```python
from build123d import *

# Parameters (mm, degrees)
SKETCH1_R            = 47
BASE_DEPTH           = 36.5
SKETCH2_W            = 38.1
SKETCH2_H            = 3.81
A_ARMS_DEPTH         = 38.1
FILLET_A_ARM_TAB_F_R = 20.32
FILLET2_R            = 50.8
SKETCH3_R            = 3.937
BOSS_EXTRUDE3_DEPTH  = 10
FILLET3_R            = 12.7
SKETCH6_R            = 3.81
TAB_HOLES_1_DEPTH    = 224.393667494
SKETCH7_R            = 3.81
TAB_HOLES_2_DEPTH    = 201.571915927
CUT_EXTRUDE2_DEPTH   = 154.791870017


with BuildPart() as part:
    # Sketch1 → Base (new body)
    with BuildSketch(Plane(origin=(0, 0, 0), x_dir=(1, 0, 0), z_dir=(0, 1, 0))):
        with BuildLine():
            Line((-80.129262367, -86.715777422), (50.125302211, -86.715777422))
            Line((50.125302211, -86.715777422), (54.750608495, -2.975412689))
            Line((54.750608495, -2.975412689), (50.125302211, 108.014745968))
            Line((50.125302211, 108.014745968), (2.575336515, 108.014745968))
            ThreePointArc((2.575336515, 108.014745968), (-20.509235608, 100.225016997), (-34.154303257, 80.041125489))
            Line((-34.154303257, 80.041125489), (-72.776330416, -60.045777422))
            Line((-72.776330416, -60.045777422), (-80.129262367, -60.045777422))
            Line((-80.129262367, -60.045777422), (-80.129262367, -86.715777422))
        make_face()
        with Locations(Location((0, 0, 0), (0, 0, 270))):
            Circle(SKETCH1_R, mode=Mode.SUBTRACT)
    extrude(amount=BASE_DEPTH)

    # Sketch2 → A-Arms (add)
    with BuildSketch(Plane(origin=(0, 36.5, 0), x_dir=(1, 0, 0), z_dir=(0, 1, 0))):
        Polygon((50.125302211, 108.014745968), (50.284076801, 104.204745968), (12.025302211, 104.204745968), (12.025302211, 108.014745968), align=None)
        Polygon((12.025302211, -82.905777422), (50.335743341, -82.905777422), (50.125302211, -86.715777422), (12.025302211, -86.715777422), align=None)
        Polygon((12.025302211, 85.154745968), (12.025302211, 81.344745968), (51.236724342, 81.344745968), (51.077949751, 85.154745968), align=None)
        Polygon((12.025302211, -60.045777422), (51.598390118, -60.045777422), (51.387948988, -63.855777422), (12.025302211, -63.855777422), align=None)
        with Locations((-61.079262367, -61.950777422)):
            Rectangle(SKETCH2_W, SKETCH2_H)
        with Locations((-61.079262367, -84.810777422)):
            Rectangle(SKETCH2_W, SKETCH2_H)
    extrude(amount=A_ARMS_DEPTH)

    # Fillet a-arm tab f
    # the kernel refuses this fillet: 20.32 mm, written as the material it takes off along each edge
    with BuildSketch(Plane(origin=(53.137354768, 74.6, 32.183090452), x_dir=(0, -1, 0), z_dir=(-0.055149831244914994, 0, 0.9984780899517313)), Plane(origin=(54.400001545, 74.6, 9.323090452), x_dir=(0, -1, 0), z_dir=(-0.055149831244913544, 0, 0.9984780899517313))) as fillet_a_arm_tab_f_piece_1:
        with BuildLine():
            CenterArc((FILLET_A_ARM_TAB_F_R, -FILLET_A_ARM_TAB_F_R), FILLET_A_ARM_TAB_F_R, 90, 90)
            Line((0, -FILLET_A_ARM_TAB_F_R), (0, 0))
            Line((0, 0), (FILLET_A_ARM_TAB_F_R, 0))
        make_face()
    extrude(amount=105.415807315, mode=Mode.SUBTRACT)
    with BuildSketch(Plane(origin=(12.025302211, 74.6, 137.515777422), x_dir=(1, 0, 0), z_dir=(0, 0, -1)), Plane(origin=(12.025302211, 74.6, -135.954745968), x_dir=(0, -1, 0), z_dir=(0, 0, 1)), Plane(origin=(-80.129262367, 74.6, 137.515777422), x_dir=(1, 0, 0), z_dir=(0, 0, -1))) as fillet_a_arm_tab_f_piece_2:
        with BuildLine():
            CenterArc((FILLET_A_ARM_TAB_F_R, FILLET_A_ARM_TAB_F_R), FILLET_A_ARM_TAB_F_R, 180, 90)
            Line((0, FILLET_A_ARM_TAB_F_R), (0, 0))
            Line((0, 0), (FILLET_A_ARM_TAB_F_R, 0))
        make_face()
    extrude(amount=105.41, mode=Mode.SUBTRACT)
    with BuildSketch(Plane(origin=(12.025302211, 74.6, 114.655777422), x_dir=(0, -1, 0), z_dir=(0, 0, -1)), Plane(origin=(12.025302211, 74.6, -53.404745968), x_dir=(0, -1, 0), z_dir=(0, 0, -1)), Plane(origin=(-42.029262367, 74.6, 32.105777422), x_dir=(0, -1, 0), z_dir=(0, 0, 1)), Plane(origin=(-42.029262367, 74.6, 114.655777422), x_dir=(-1, 0, 0), z_dir=(0, 0, -1)), Plane(origin=(-80.129262367, 74.6, 9.245777422), x_dir=(1, 0, 0), z_dir=(0, 0, 1))) as fillet_a_arm_tab_f_piece_3:
        with BuildLine():
            CenterArc((FILLET_A_ARM_TAB_F_R, -FILLET_A_ARM_TAB_F_R), FILLET_A_ARM_TAB_F_R, 90, 90)
            Line((0, -FILLET_A_ARM_TAB_F_R), (0, 0))
            Line((0, 0), (FILLET_A_ARM_TAB_F_R, 0))
        make_face()
    extrude(amount=105.41, mode=Mode.SUBTRACT)
    with BuildSketch(Plane(origin=(53.351883028, 74.6, -30.588799481), x_dir=(0, -1, 0), z_dir=(-0.04163698201983484, 0, -0.9991328048504263)), Plane(origin=(48.010143525, 74.6, -158.770692454), x_dir=(-0.9991328048504262, 0, 0.04163698201983669), z_dir=(0.0416369820198367, 0, 0.9991328048504262))) as fillet_a_arm_tab_f_piece_4:
        with BuildLine():
            CenterArc((FILLET_A_ARM_TAB_F_R, FILLET_A_ARM_TAB_F_R), FILLET_A_ARM_TAB_F_R, 180, 90)
            Line((0, FILLET_A_ARM_TAB_F_R), (0, 0))
            Line((0, 0), (FILLET_A_ARM_TAB_F_R, 0))
        make_face()
    extrude(amount=105.413306881, mode=Mode.SUBTRACT)

    # Fillet2
    # the kernel refuses this fillet: 50.8 mm, written as the material it takes off along each edge
    with BuildSketch(Plane(origin=(54.750608495, -6.153313098, 2.975412689), x_dir=(-0.05514983124491408, 0, 0.9984780899517313), z_dir=(0, 1, 0))) as fillet2_piece_1:
        with BuildLine():
            CenterArc((FILLET2_R * 0.0484512842399, -FILLET2_R), FILLET2_R, 90, 5.547769732)
            Line((-FILLET2_R * 0.0482243356174, -FILLET2_R * 0.00468405793677), (0, 0))
            Line((0, 0), (FILLET2_R * 0.0484512842399, 0))
        make_face()
    extrude(amount=48.806626197, mode=Mode.SUBTRACT)

    # Sketch3 → Boss-Extrude3 (add)
    with BuildSketch(Plane(origin=(0, 1, 0), x_dir=(-1, 0, 0), z_dir=(0, -1, 0))):
        with BuildLine():
            Line((42.093323872, 51.245308907), (62.210800727, -21.723285296))
            Line((62.210800727, -21.723285296), (72.188506448, -18.972426984))
            ThreePointArc((72.188506448, -18.972426984), (77.618129068, -10.048878041), (69.039031874, -4.089883254))
            ThreePointArc((69.039031874, -4.089883254), (65.518990894, -3.323443269), (63.392280792, -0.415656673))
            Line((63.392280792, -0.415656673), (54.014483076, 33.598783658))
            ThreePointArc((54.014483076, 33.598783658), (54.320283062, 37.122596493), (56.852004495, 39.592648541))
            ThreePointArc((56.852004495, 39.592648541), (60.937845875, 49.122693965), (51.737082765, 53.904097917))
            Line((51.737082765, 53.904097917), (42.093323872, 51.245308907))
        make_face()
        with Locations(Location((70.163230544, -11.62649903, 0), (0, 0, 90))):
            Circle(SKETCH3_R, mode=Mode.SUBTRACT)
        with Locations(Location((53.76235867, 46.558169963, 0), (0, 0, 90))):
            Circle(SKETCH3_R, mode=Mode.SUBTRACT)
    extrude(amount=-BOSS_EXTRUDE3_DEPTH)

    # Fillet3
    # the kernel refuses this fillet: 12.7 mm, written as the material it adds along each edge
    with BuildSketch(Plane(origin=(-42.093323872, 1, -51.245308907), x_dir=(0.26578423939908447, 0, -0.9640325399523867), z_dir=(0, 1, 0))) as fillet3_piece_1:
        with BuildLine():
            CenterArc((12.520298407, 12.7), FILLET3_R, 187.62557017, 82.37442983)
            Line((-0.067388097, 11.014725997), (-1.326156748, 10.846198597))
            ThreePointArc((-1.326156748, 10.846198597), (-1.27, 10.003561596), (-1.27, 0))
            Line((-1.27, 0), (0, -1.27))
            Line((0, -1.27), (12.520298407, -1.27))
            Line((12.520298407, -1.27), (12.520298407, 0))
        make_face()
    extrude(amount=10)
    with BuildSketch(Plane(origin=(-62.210800727, 1, 21.723285296), x_dir=(-0.26578423939908535, 0, 0.9640325399523866), z_dir=(0, 1, 0))) as fillet3_piece_2:
        with BuildLine():
            CenterArc((12.563650525, -12.7), FILLET3_R, 90, 83.358813764)
            Line((-0.051131053, -11.231229858), (-1.312609211, -11.084352844))
            ThreePointArc((-1.312609211, -11.084352844), (-1.27, -10.349967773), (-1.27, 0))
            Line((-1.27, 0), (0, 1.27))
            Line((0, 1.27), (12.563650525, 1.27))
            Line((12.563650525, 1.27), (12.563650525, 0))
        make_face()
    extrude(amount=10)

    # Sketch6 → Tab Holes 1 (cut, through all)
    with BuildSketch(Plane(origin=(0, 0, -108.014745968), x_dir=(-1, 0, 0), z_dir=(0, 0, -1))):
        with Locations((-31.067038594, 61.859754489)):
            Circle(SKETCH6_R)
    extrude(amount=-TAB_HOLES_1_DEPTH, mode=Mode.SUBTRACT)

    # Sketch7 → Tab Holes 2 (cut, through all)
    with BuildSketch(Plane(origin=(0, 0, 60.045777422), x_dir=(-1, 0, 0), z_dir=(0, 0, -1))):
        with Locations((61.079262367, 61.860273667)):
            Circle(SKETCH7_R)
    extrude(amount=-TAB_HOLES_2_DEPTH, mode=Mode.SUBTRACT)

    # Sketch8 → Cut-Extrude2 (cut, through all)
    with BuildSketch(Plane(origin=(0, 0, 0), x_dir=(1, 0, 0), z_dir=(0, 1, 0))):
        with BuildLine():
            Line((-29.257017954, 78.690941553), (-42.752390199, 29.741545559))
            ThreePointArc((-42.752390199, 29.741545559), (6.494009323, 51.673535228), (48.782168121, 18.238050153))
            Line((48.782168121, 18.238050153), (46.36401462, 76.264745968))
            Line((46.36401462, 76.264745968), (6.945302211, 76.264745968))
            Line((6.945302211, 76.264745968), (6.945302211, 90.234745968))
            Line((6.945302211, 90.234745968), (45.781841123, 90.234745968))
            Line((45.781841123, 90.234745968), (45.41136708, 99.124745968))
            Line((45.41136708, 99.124745968), (6.945302211, 99.124745968))
            Line((6.945302211, 99.124745968), (6.945302211, 102.934745968))
            Line((6.945302211, 102.934745968), (2.575336515, 102.934745968))
            ThreePointArc((2.575336515, 102.934745968), (-17.431292658, 96.183647526), (-29.257017954, 78.690941553))
        make_face()
        with BuildLine():
            Line((-75.049262367, -77.825777422), (-36.949262367, -77.825777422))
            Line((-36.949262367, -77.825777422), (-36.949262367, -81.635777422))
            Line((-36.949262367, -81.635777422), (6.945302211, -81.635777422))
            Line((6.945302211, -81.635777422), (6.945302211, -77.825777422))
            Line((6.945302211, -77.825777422), (45.528588426, -77.825777422))
            Line((45.528588426, -77.825777422), (46.019617728, -68.935777422))
            Line((46.019617728, -68.935777422), (6.945302211, -68.935777422))
            Line((6.945302211, -68.935777422), (6.945302211, -54.965777422))
            Line((6.945302211, -54.965777422), (46.791235203, -54.965777422))
            Line((46.791235203, -54.965777422), (48.826411186, -18.119270701))
            ThreePointArc((48.826411186, -18.119270701), (-7.410849482, -51.550031134), (-51.953259135, -3.631152049))
            Line((-51.953259135, -3.631152049), (-66.106240279, -54.965777422))
            Line((-66.106240279, -54.965777422), (-36.949262367, -54.965777422))
            Line((-36.949262367, -54.965777422), (-36.949262367, -68.935777422))
            Line((-36.949262367, -68.935777422), (-75.049262367, -68.935777422))
            Line((-75.049262367, -68.935777422), (-75.049262367, -77.825777422))
        make_face()
    extrude(amount=CUT_EXTRUDE2_DEPTH, mode=Mode.SUBTRACT)


solid = part.part
```
Geometry check sheet. Reference: the model listing, model coordinates, mm. A direction names the side the tool comes from. Coordinates: 2 decimals unless noted, no trailing zeros. Order: outer loops, then holes, each group sorted by start corner. A loop starts at its lowest first (then second) coordinate and runs counter-clockwise, first axis right, second up. Notation, with made-up numbers: M -36.5,2 L 18.5,2 A23 cw 18.5,30 Z; hole C 22,17 d6. An arc over 180 degrees is marked long. Answer as a JSON object with one key per item and string values.
Q1. Cross-section at D-D on z = -13. Record the cut outline in (x, y).
Results are:
{"outline": "M -59.69,1 L -52.64,1 L -52.64,0 L -45.17,0 L -45.17,36.5 L -52.64,36.5 L -52.64,11 L -59.69,11 Z; M 45.17,0 L 54.08,0 L 54.08,36.5 L 45.17,36.5 Z"}
Q2. Depth check by flat-ended pin: pin 1 Ø5 at (y, z) = (11, 56.5) entering from -X; pin 2 Ø19 at (x, y) = (-61, 47) entering from -Z; pin 3 Ø11 at (y, z) = (25.5, -81.5) entering from -X; pin 4 Ø6.5 at (x, z) = (-70.16, 11.63) entering from -Y. Enter the tip coordinate at first touch or a pass-through.
Results are:
{"pin 1": "stops at x = -72.49", "pin 2": "stops at z = 60.05", "pin 3": "stops at x = -35.27", "pin 4": "passes through"}
Q3. Tool access check on faces 4 (the flat face through (31, 55, -104.205)), 5 (the flat face through (-42.029, 45, 62)), 6 (the flat face through (-57, 1, -15)). Record the directions out of +Z, -Z, +X, -X, +Y, -Y that give a thin tool (end or side, any length) a straight path to the whole face; none if there is none.
Results are:
{"face 4": "+X, -X, +Y", "face 5": "+Z, -Z, +Y", "face 6": "-Z, -X, -Y"}
Q4. Cross-section at B-B on y = 70.5. Record the cut outline in (x, z), and give its area (3 significant figures).
Results are:
{"outline": "M -72.05,60.05 L -50.11,60.05 L -50.11,63.86 L -72.05,63.86 Z; M -72.05,82.91 L -50.11,82.91 L -50.11,86.72 L -72.05,86.72 Z; M 20.11,-108.01 L 42.04,-108.01 L 42.2,-104.2 L 20.11,-104.2 Z; M 20.11,-85.15 L 42.99,-85.15 L 43.15,-81.34 L 20.11,-81.34 Z; M 20.11,60.05 L 43.51,60.05 L 43.3,63.86 L 20.11,63.86 Z; M 20.11,82.91 L 42.24,82.91 L 42.03,86.72 L 20.11,86.72 Z", "area": "511 mm²"}
Q5. Cross-section at C-C on x = 0. Record the cut outline in (y, z), and give its area (3 significant figures).
Results are:
{"outline": "M 0,-107.93 L 36.5,-107.93 L 36.5,-102.83 L 0,-102.83 Z; M 0,-52.08 L 36.5,-52.08 L 36.5,-47 L 0,-47 Z; M 0,47 L 36.5,47 L 36.5,52.08 L 0,52.08 Z; M 0,81.64 L 36.5,81.64 L 36.5,86.72 L 0,86.72 Z", "area": "742 mm²"}
Q6. Release check for a two-part mould opening along X. For faces 1 (the flat face through (-58.77, 5.93, -16.35)), 2 (the flat face through (32, 55, 63.856)), 3 (the cylindrical face through (17.632, 68.295, 61.977)) record: released by +X, released by -X, zero draft, split by the parting line, or undercut.
Results are:
{"face 1": "released by -X", "face 2": "zero draft", "face 3": "undercut"}
Q7. Scan lines: line 1 (Z direction, x = 28, y = 68); line 2 (Z direction, x = 19.5, y = 5); line 3 (Z direction, x = -3.5, y = 22). Record each from-to range of solid material in increasing order.
Results are:
{"line 1": "z = -108.01 to -104.2, -85.15 to -81.34, 60.05 to 63.86, 82.91 to 86.72", "line 2": "z = -108.01 to -99.12, -90.23 to -76.26, -48.29 to -42.76, 42.76 to 48.29, 54.97 to 68.94, 77.83 to 86.72", "line 3": "z = -107.53 to -102.37, -51.96 to -46.87, 46.87 to 51.96, 81.64 to 86.72"}
Q8. Cross-section at A-A on z = 38. Record the cut outline in (x, y).
Results are:
{"outline": "M -66.7,0 L -61.43,0 L -61.43,36.5 L -66.7,36.5 Z; M -35.61,0 L -27.66,0 L -27.66,36.5 L -35.61,36.5 Z; M 27.66,0 L 35.61,0 L 35.61,36.5 L 27.66,36.5 Z; M 47.73,0 L 52.82,0 L 52.82,36.5 L 47.73,36.5 Z"}
